Input: part model. Units: mm. Frame: model coordinates. Face numbers are marked on the shaded views. Coordinates: 2 decimals unless noted, no trailing zeros. Order: outer loops, then holes, each group sorted by start corner. A loop starts at its lowest first (then second) coordinate and runs counter-clockwise, first axis right, second up. Notation, with made-up numbers: M -10.5,2 L 32.5,2 A25 ccw 32.5,32 Z; hole C -3.5,45.5 d1. An arc over 180 degrees is marked long. One line per item, written item: value.
```python
from build123d import *

# Parameters (mm, degrees)
SKETCH1_R           = 10
BOSS_EXTRUDE1_DEPTH = 1.8
CUT_EXTRUDE1_START  = -0.9
SKETCH2_R           = 10
SKETCH2_R_2         = 8
CUT_EXTRUDE1_DEPTH  = 0.9
FILLET2_R           = 2
SKETCH3_R           = 1.75
CUT_EXTRUDE2_DEPTH  = 0.9


with BuildPart() as part:
    # Sketch1 → Boss-Extrude1 (new body)
    with BuildSketch(Plane(origin=(0, 0, 0), x_dir=(0, 1, 0), z_dir=(0, 0, 1))):
        with Locations(Location((0, 0, 0), (0, 0, 270))):
            Circle(SKETCH1_R)
    extrude(amount=BOSS_EXTRUDE1_DEPTH)

    # Sketch2 → Cut-Extrude1 (cut)
    with BuildSketch(Plane.XY.offset(1.8).offset(CUT_EXTRUDE1_START)):
        Circle(SKETCH2_R)
        Circle(SKETCH2_R_2, mode=Mode.SUBTRACT)
    extrude(amount=CUT_EXTRUDE1_DEPTH, mode=Mode.SUBTRACT)

    # Fillet2
    # the kernel refuses this fillet: 2 mm, written as the material it adds along each edge
    with BuildSketch(Plane(origin=(0, 0, 0.9), x_dir=(1, 0, 0), z_dir=(0, -1, 0))) as fillet2_piece_1:
        with BuildLine():
            CenterArc((9.670329309, 2), FILLET2_R, 213.367012969, 56.632987031)
            Line((8, 0.9), (7.966593414, 0.878))
            ThreePointArc((7.966593414, 0.878), (7.96, 0.45), (7.96, 0))
            Line((7.96, 0), (8, -0.04))
            Line((8, -0.04), (9.670329309, -0.04))
            Line((9.670329309, -0.04), (9.670329309, 0))
        make_face()
    revolve(axis=Axis((0, 0, 0.9), (0, 0, 1)))

    # Sketch3 → Cut-Extrude2 (cut)
    with BuildSketch(Plane.XY.offset(1.8)):
        Circle(SKETCH3_R)
    extrude(amount=-CUT_EXTRUDE2_DEPTH, mode=Mode.SUBTRACT)


solid = part.part
```
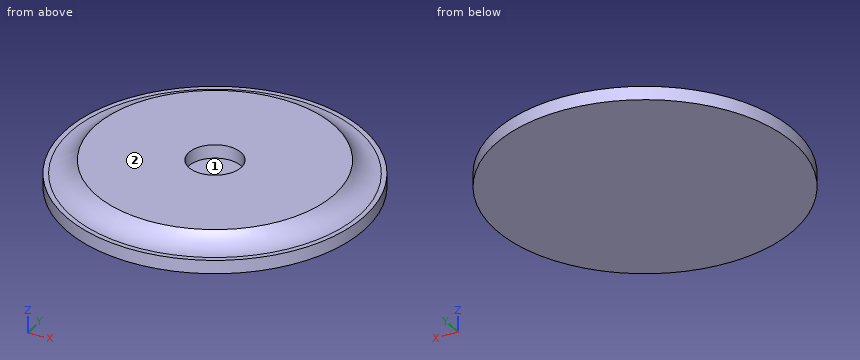
(1) Draft query along X for the marked faces 1 and 2. Return one class per face: released by +X, released by -X, zero draft, split by the parting line, or undercut.
Data:
face 1: undercut
face 2: zero draft
(2) Ray query, line 1 (Y direction, x = 0, z = 1.65); line 2 (Y direction, x = 0, z = 1.4); line 3 (Y direction, x = 8.25, z = 0.65). Return the intervals inside material, ascending. Write a range as from..to.
Data:
line 1: y = -8.11..-1.75, 1.75..8.11
line 2: y = -8.35..-1.75, 1.75..8.35
line 3: y = -5.65..5.65
(3) Cut plane A-A on x = 0. Output: boundary loops of the cut face in (y, z).
Data:
outline: M -10,0 L 10,0 L 10,0.9 L 9.67,0.9 A2 cw 8,1.8 L 1.75,1.8 L 1.75,0.9 L -1.75,0.9 L -1.75,1.8 L -8,1.8 A2 cw -9.67,0.9 L -10,0.9 Z
(4) First-contact query: pin 1 (1.8 mm diameter, centred on x = 0.5, y = 0, fed in from +Z). Flat tip, straight axial feed; report the tip coordinate or a pass-through.
Data:
pin 1: stops at z = 0.9
(5) Cut plane C-C on z = 1.25. Output: boundary loops of the cut face in (x, y).
Data:
outline: C 0,0 d17.08; hole C 0,0 d3.5
